Job drawing, mm, ordinate dimensions from the low corner. One solid piece. A direction names the side the tool comes from. Round coordinates to 2 decimals unless told otherwise and drop trailing zeros. Write each loop counter-clockwise with the first axis right and the second up, starting at its lowest first coordinate (ties: lowest second). Pieces come first, ordered by that corner, then holes. Notation, with made-up numbers: M 65,-33.75 L 86,-33.75 A24 ccw 86,1.25 Z; hole C 2.5,87.25 d7. An arc over 180 degrees is marked long. Answer as a JSON object with one key per item and string values. Group by question number.
1. Drill centre lines: line 1 (Y direction, x = 65, z = 4.8); line 2 (Y direction, x = 81.5, z = 6.75); line 3 (Z direction, x = 62, y = 34). Where is each one in solid material? Low to high. Write a range as from..to.
2. Drop flat-ended pins along their axis: pin 1 (23.5 mm diameter, centred on x = 55.5, y = 48.5, fed in from -Z); pin 2 (3 mm diameter, centred on x = 86, y = 9, fed in from -Z); pin 3 (4.5 mm diameter, centred on x = 74, z = 1.5, fed in from +Y). Give the stop position or say it passes through.
3. Which spindle directions (+Z, -Z, +X, -X, +Y, -Y) get a long thin tool onto all of the face, cutting with end or side? Do the marked faces 1 and 2. Say none if no direction does.
4. Band-saw the part on A-A, the plane z = 1.75. Write the cut outline in (x, y).
5. Band-saw the part on D-D, the plane x = 17. Write the cut outline in (y, z), plus the area to 3 significant figures.
6. Band-saw the part on C-C, the plane y = 59. Write the cut outline in (x, z).
7. Band-saw the part on B-B, the plane x = 50. Write the cut outline in (y, z), plus the area to 3 significant figures.
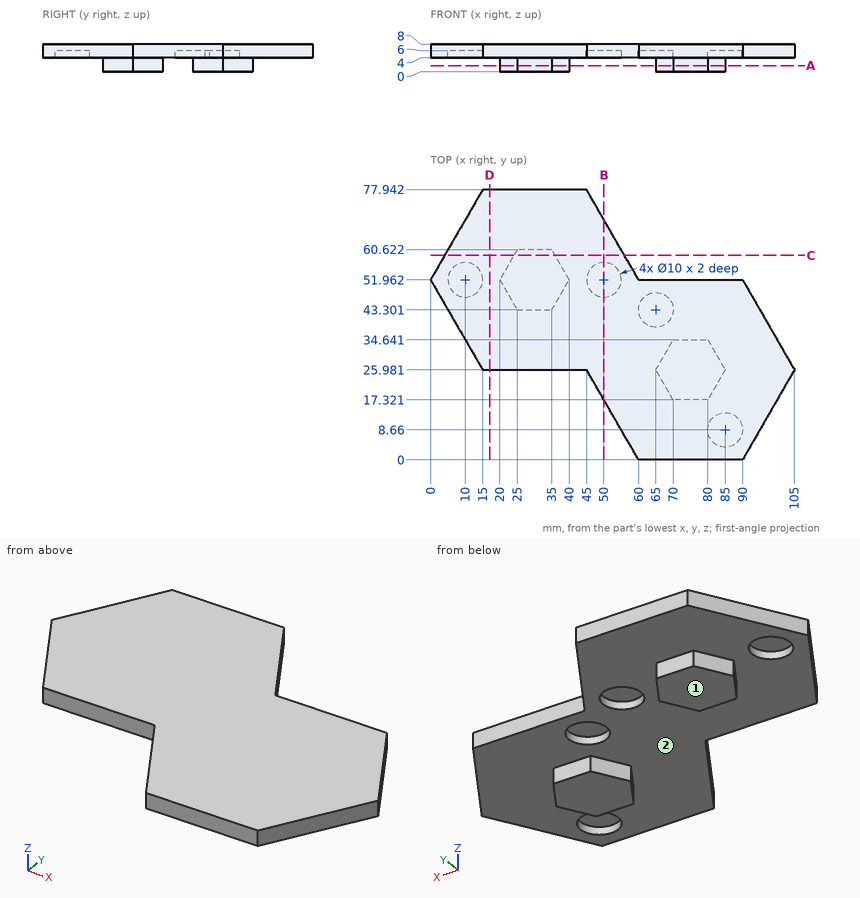
Worked answers:
{
 "1": {"line 1": "y = 0..38.3, 48.3..51.96", "line 2": "y = 0..51.96", "line 3": "z = 4..8"},
 "2": {"pin 1": "stops at z = 4", "pin 2": "stops at z = 6", "pin 3": "stops at y = 34.64"},
 "3": {"face 1": "-Z, +X, -X, +Y, -Y", "face 2": "-Z"},
 "4": {"outline": "M 20,51.96 L 25,43.3 L 35,43.3 L 40,51.96 L 35,60.62 L 25,60.62 Z; M 65,25.98 L 70,17.32 L 80,17.32 L 85,25.98 L 80,34.64 L 70,34.64 Z"},
 "5": {"outline": "M 25.98,4 L 77.94,4 L 77.94,8 L 25.98,8 Z", "area": "208 mm^2"},
 "6": {"outline": "M 4.06,4 L 24.06,4 L 24.06,0 L 35.94,0 L 35.94,4 L 55.94,4 L 55.94,8 L 4.06,8 Z"},
 "7": {"outline": "M 17.32,4 L 46.96,4 L 46.96,6 L 56.96,6 L 56.96,4 L 69.28,4 L 69.28,8 L 17.32,8 Z", "area": "188 mm^2"}
}
